Source: CAD feature listing. Evaluate the final solid. Frame: model axes, mm. A direction names the side the tool comes from. Give positions to 0.01 mm unless a question says otherwise; leave off trailing zeros. Loops run counter-clockwise (first coordinate to the right, second up) from the corner with the lowest first, then second, coordinate; pieces in that order, holes last. Notation, with made-up numbers: M 56,-28.5 L 66,-28.5 A6 cw 66,-23.5 Z; hole C 64.25,-24.75 d11. An arc over 180 degrees is marked long. Put each result on its own line as item: value.
from build123d import *

# Parameters (mm, degrees)
SKETCH1_W                                       = 180
SKETCH1_H                                       = 150
BOSS_EXTRUDE1_DEPTH                             = 5
CSK_FOR_M2_FLAT_HEAD_MACHINE_SCREW1_D           = 2.4
CSK_FOR_M2_FLAT_HEAD_MACHINE_SCREW1_CSINK_D     = 4.4
CSK_FOR_M2_FLAT_HEAD_MACHINE_SCREW1_CSINK_ANGLE = 90
SKETCH5_R                                       = 21
BOSS_EXTRUDE3_DEPTH                             = 5
SKETCH6_R                                       = 2.5
BOSS_EXTRUDE4_DEPTH                             = 60
F_1_0MM_DOWEL_HOLE1_OUTLINE_R                   = 0.5
F_1_0MM_DOWEL_HOLE1_DEPTH                       = 5


# Read off the part's stored shape, not the designer's step: Ø1.0mm Dowel Hole1
with BuildPart() as part:
    # Sketch1 → Boss-Extrude1 (new body)
    with BuildSketch(Plane(origin=(0, 0, 0), x_dir=(1, 0, 0), z_dir=(0, 1, 0))):
        Rectangle(SKETCH1_W, SKETCH1_H)
    extrude(amount=BOSS_EXTRUDE1_DEPTH)

    # CSK for M2 Flat Head Machine Screw1 (through all)
    with Locations(Plane(origin=(-82, 5, -67), x_dir=(0, 0, 1), z_dir=(0, 1, 0))):
        with Locations((0, 0), (67, 0), (134, 0), (134, 82), (134, 164), (67, 164), (0, 164), (0, 82)):
            CounterSinkHole(CSK_FOR_M2_FLAT_HEAD_MACHINE_SCREW1_D / 2, CSK_FOR_M2_FLAT_HEAD_MACHINE_SCREW1_CSINK_D / 2, counter_sink_angle=CSK_FOR_M2_FLAT_HEAD_MACHINE_SCREW1_CSINK_ANGLE)

    # Sketch5 → Boss-Extrude3 (add)
    with BuildSketch(Plane(origin=(0, 5, 0), x_dir=(1, 0, 0), z_dir=(0, 1, 0))):
        with Locations(Location((-60, -45, 0), (0, 0, 270))):
            Circle(SKETCH5_R)
        with Locations(Location((-60, 45, 0), (0, 0, 270))):
            Circle(SKETCH5_R)
        with Locations(Location((60, 45, 0), (0, 0, 270))):
            Circle(SKETCH5_R)
        with Locations(Location((60, -45, 0), (0, 0, 270))):
            Circle(SKETCH5_R)
    extrude(amount=BOSS_EXTRUDE3_DEPTH)

    # Sketch6 → Boss-Extrude4 (add)
    with BuildSketch(Plane(origin=(0, 0, 0), x_dir=(-1, 0, 0), z_dir=(0, -1, 0))):
        with Locations(Location((60, 48, 0), (0, 0, 270))):
            Circle(SKETCH6_R)
        with Locations(Location((60, -49, 0), (0, 0, 270))):
            Circle(SKETCH6_R)
        with Locations(Location((-37, 48, 0), (0, 0, 270))):
            Circle(SKETCH6_R)
        with Locations(Location((-37, -49, 0), (0, 0, 270))):
            Circle(SKETCH6_R)
    extrude(amount=BOSS_EXTRUDE4_DEPTH)

    # Ø1.0mm Dowel Hole1 outline → Ø1.0mm Dowel Hole1 (cut)
    with BuildSketch(Plane(origin=(0, 0, 0), x_dir=(1, 0, 0), z_dir=(0, 1, 0))):
        with Locations((37, -49)):
            Circle(F_1_0MM_DOWEL_HOLE1_OUTLINE_R)
    extrude(amount=F_1_0MM_DOWEL_HOLE1_DEPTH, mode=Mode.SUBTRACT)

    # 1.0mm Dowel Hole1 2 outline → 1.0mm Dowel Hole1 2 (revolve, cut)
    with BuildSketch(Plane(origin=(37, 0, -48), x_dir=(1, 0, 0), z_dir=(0, 0, 1))):
        Polygon((0.5, -30), (0, -29.69956969), (0, -60), (0.5, -60), align=None)
    revolve(axis=Axis((37, 0, -48), (0, 1, 0)), mode=Mode.SUBTRACT)

    # 1.0mm Dowel Hole1 3 outline → 1.0mm Dowel Hole1 3 (revolve, cut)
    with BuildSketch(Plane(origin=(-60, 0, 49), x_dir=(1, 0, 0), z_dir=(0, 0, 1))):
        Polygon((0.5, -30), (0, -29.69956969), (0, -60), (0.5, -60), align=None)
    revolve(axis=Axis((-60, 0, 49), (0, 1, 0)), mode=Mode.SUBTRACT)

    # 1.0mm Dowel Hole1 4 outline → 1.0mm Dowel Hole1 4 (revolve, cut)
    with BuildSketch(Plane(origin=(-60, 0, -48), x_dir=(1, 0, 0), z_dir=(0, 0, 1))):
        Polygon((0.5, -30), (0, -29.69956969), (0, -60), (0.5, -60), align=None)
    revolve(axis=Axis((-60, 0, -48), (0, 1, 0)), mode=Mode.SUBTRACT)


solid = part.part
1. Draft query along Z for faces 4 (the cylindrical face through (37.96, -29.58, -45.69)), 5 (the flat face through (-1, 2, -75)), 6 (the flat face through (-90, 2, 1)). Return one class per face: pulls with the +Z half, pulls with the -Z half, needs draft (parallel to the pull), parting line crosses it, or undercut.
Found:
face 4: undercut
face 5: pulls with the -Z half
face 6: needs draft
2. Section query C-C (y = -27). Output: boundary loops of the cut face in (x, z), plus the area to 3 significant figures.
Found:
outline: C -60,-48 d5; C -60,49 d5; C 37,-48 d5; C 37,49 d5
area: 78.5 mm^2
3. Section query B-B (x = 60). Output: boundary loops of the cut face in (y, z).
Found:
outline: M 0,-75 L 5,-75 L 5,-66 L 10,-66 L 10,-24 L 5,-24 L 5,24 L 10,24 L 10,66 L 5,66 L 5,75 L 0,75 Z
4. Access query for faces 1 (the flat face through (-60, 10, 45)), 2 (the cylindrical face through (-59.04, -29.58, -45.69)), 3 (the cylindrical face through (80.82, 7.46, -47.73)). Directions: +Z, -Z, +X, -X, +Y, -Y. A direction counts if a zero-diameter tool reaches every point of the face in a straight line with its end or side. Return the directions, or none.
Found:
face 1: +Z, -Z, +X, -X, +Y
face 2: -Y
face 3: +Y
5. Section query D-D (z = -9.5). Output: boundary loops of the cut face in (x, y), plus the area to 3 significant figures.
Found:
outline: M -90,0 L 90,0 L 90,5 L -90,5 Z
area: 900 mm^2
6. Section query A-A (y = -44.5). Output: boundary loops of the cut face in (x, z), plus the area to 3 significant figures.
Found:
outline: C -60,-48 d5; C -60,49 d5; C 37,-48 d5; C 37,49 d5; hole C -60,-48 d1; hole C -60,49 d1; hole C 37,-48 d1
area: 76.2 mm^2
7. Material intervals for line 1 (X direction, y = 2.35, z = -67); line 2 (X direction, y = 1.75, z = 0); line 3 (Z direction, x = 82, y = 1), sorted ascending. Write a range as from..to.
Found:
line 1: -90..-83.2, -80.8..-1.2, 1.2..80.8, 83.2..90
line 2: -90..-83.2, -80.8..80.8, 83.2..90
line 3: -75..-68.2, -65.8..-1.2, 1.2..65.8, 68.2..75
8. Contact query for flat-ended pins moving along their axis: P1, Ø3, axis at x = 0, z = 67, coming from the -Y side; P2, Ø3, axis at x = -82, z = 0, coming from the +Y side; P3, Ø8, axis at y = -26.5, z = -48.5, coming from the +X side. Output: stop coordinate, or through.
Found:
P1: y = 0
P2: y = 4.3
P3: x = 39.5
